Check sheet for the modelled part. Datum: model origin and axes. Units: mm. Face numbers are marked on the shaded views. Coordinates: 2 decimals unless noted, no trailing zeros. Order: outer loops, then holes, each group sorted by start corner. A loop starts at its lowest first (then second) coordinate and runs counter-clockwise, first axis right, second up. Notation, with made-up numbers: (5, -30) -> (57, -30) arc R17 ccw to (57, -22) -> close; hole circle Ø8 at (25, 87.5). An arc over 180 degrees is marked (long way). Put each result on its own line as item: value. Start each with the question number.
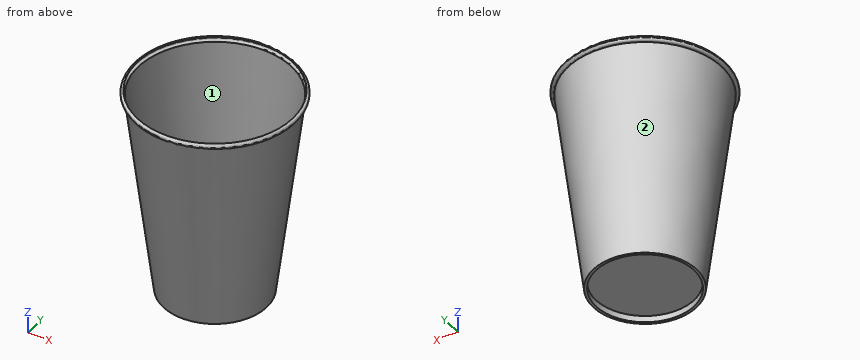
```python
from build123d import *

# Parameters (mm, degrees)
F2_R     = 25.4
F0_R     = 38.1
F3_R     = 24.13
F5_DEPTH = 3.175
F6_R     = 39.37
F7_DEPTH = 2.54
F8_R     = 1.26999
F9_T     = -0.254


# Not quite as in the source:
# - a fillet or chamfer is up to 0.001 mm smaller than in the source, because OpenCascade refuses the exact size
# - a shell that OpenCascade refuses in one call is made with other operations: the cavity is built on its own and cut out


with BuildPart() as f4:
    # F2 (on offset) → F4 section 0
    with BuildSketch(Plane.XY.offset(-101.6)):
        Circle(F2_R)
    # F0 (on Top) → F4 section 1
    with BuildSketch(Plane.XY):
        Circle(F0_R)
    loft()

    # F3 (on offset) → F5 (cut)
    with BuildSketch(Plane.XY.offset(-101.6)):
        Circle(F3_R)
    extrude(amount=F5_DEPTH, mode=Mode.SUBTRACT)

    # F6 (on Top) → F7 (join)
    with BuildSketch(Plane.XY):
        Circle(F6_R)
    extrude(amount=-F7_DEPTH)

    # F8 (radius 1.27 in the source; OpenCascade refuses exactly that, so slightly less here)
    f8_edges = [f4.edges().sort_by_distance(p)[0] for p in [
        (-39.37, 0, -2.54),
        (-39.37, 0, 0),
    ]]
    fillet(f8_edges, radius=F8_R)

    # F9: a shell. OpenCascade refuses it in one call, so the cavity is built on its own and cut out:
    # the body offset inwards by the wall thickness, plus a prism from it out through each open face.
    f9_core = offset(f4.part, amount=F9_T, kind=Kind.INTERSECTION, mode=Mode.PRIVATE)
    f9_exits = [f9_core.faces().sort_by_distance(p)[0] for p in [
        (0, 0, -0.254),
    ]]
    add(f9_core, mode=Mode.SUBTRACT)
    extrude(f9_exits, amount=-F9_T, mode=Mode.SUBTRACT)


solid = f4.part
```
1) Sectioned sample at B-B (z = -24.5). Record the boundary of the cut face in (x, y) (1 decimal), plus the area to 3 significant figures.
2) Mould release check, pull along X, two halves, no side actions. Record for the marked faces 1 and 2: +X half, -X half, draft (parallel to the pull), parting line (faces both ways), or undercut.
3) Gauge pin test, flat ends, axial feed: pin 1 (3 mm diameter, centred on y = -13.5, z = -13.5, fed in from +X); pin 2 (10 mm diameter, centred on y = -25, z = -83.5, fed in from -X); pin 3 (6 mm diameter, centred on x = 18, y = -1, fed in from +Z). Record the tip position at first contact, or that the pin passes through.
4) Scan lines: line 1 along Y through (x, z) = (0, -1.3); line 2 along X through (y, z) = (-15, -91); line 3 along Y through (x, z) = (-4, -50.5). Record each from-to range of solid material in increasing order. Write a range as [from, to].
5) Sectioned sample at C-C (z = -13). Record the boundary of the cut face in (x, y) (3 decimals), plus the area to 3 significant figures.
Entries:
1. outline: circle Ø70.1 at (0, 0); hole circle Ø69.6 at (0, 0)
1. area: 56.1 mm2
2. face 1: undercut
2. face 2: parting line
3. pin 1: stops at x = 34.41
3. pin 2: stops at x = -19.19
3. pin 3: stops at z = -98.17
4. line 1: y = [-39.37, -39.12], [39.12, 39.37]
4. line 2: x = [-22.12, -21.81], [21.81, 22.12]
4. line 3: y = [-31.53, -31.28], [31.28, 31.53]
5. outline: circle Ø72.95 at (0, 0); hole circle Ø72.438 at (0, 0)
5. area: 58.5 mm2
